Read the model definition and answer for the solid it produces. Units are mm, in the model's axes. A direction names the side the tool comes from. Coordinates: 2 decimals unless noted, no trailing zeros. Loops run counter-clockwise (first coordinate to the right, second up) from the corner with the lowest first, then second, coordinate; pieces in that order, holes last.
Q1. The mould has two halves that part along Z. Classify faces 1 (the face through (0, 0, 15)), 2 (the face through (-22.465, -1.617, -0.67)), 3 (the face through (0, -0.75, 9)), 4 (the face through (0, 9, -0.75)): pulls with the +Z half, pulls with the -Z half, needs draft (parallel to the pull), parting line crosses it, or undercut.
Q2. Which of the six approach directions +Z, -Z, +X, -X, +Y, -Y give full straight-line access (tool end or side, diameter ignored) to faces 5 (the face through (0.28, -6.6, 5.55)), 6 (the face through (0, -0.75, -9)), 7 (the face through (0.28, 5.54, 6.61))?
Q3. Section C-C (z = -3.5) is taken. Give the vertices of the cut face in (x, y), then the cut area to 3 significant figures.
Q4. Straight lines are drawn through the part: line 1 (Z direction, x = 12, y = -10.5); line 2 (Z direction, x = -9.5, y = -5.5); line 3 (Y direction, x = 1, z = 8.5). For each, find the intervals that lie inside material, in ascending order.
Q5. Flat-ended cylindrical pins translate along their axes: P1, Ø1.5, axis at y = 9.5, z = -7, coming from the +X side; P2, Ø6.5, axis at x = 1.5, y = -9, coming from the -Z side; P3, Ø4, axis at x = 3.5, y = -6, coming from the +Z side; P4, Ø14, axis at x = 3.5, y = 9, coming from the +Z side. Find the tip coordinate at first contact, or state that the pin passes through.
Q6. Section A-A (y = -3.75) is taken. Give the vertices of the cut face in (x, z), then the cut area to 3 significant figures.
Q7. Section D-D (z = -12) is taken. Give the vertices of the cut face in (x, y), then the cut area to 3 significant figures.
from build123d import *

# Parameters (mm, degrees)
F0_W          = 40
F0_H          = 15
F3_DEPTH      = 40.001
F4_R          = 1.75
F4_R_2        = 0.75
F6_DEPTH      = 5
F6_DEPTH_BACK = 80


with BuildPart() as f1:
    # F0 (on Top) → F1 (revolve)
    with BuildSketch(Plane.XY):
        with Locations((0, 7.5)):
            Rectangle(F0_W, F0_H)
    revolve(axis=Axis((0, 0, 0), (1, 0, 0)))

    # F2 (on face) → F3 (cut, through all)
    with BuildSketch(Plane.YZ.offset(20)):
        with BuildLine():
            ThreePointArc((1.651475323, -0.578903496), (1.7251930059, -0.2936138491), (1.75, 0))
            ThreePointArc((1.75, 0), (1.7236043316, 0.3028004429), (1.6452135906, 0.5964664628))
            ThreePointArc((1.6452135906, 0.5964664628), (1.6150017407, 0.6739950872), (1.5811388301, 0.75))
            ThreePointArc((1.5811388301, 0.75), (1.2374368671, 1.2374368671), (0.75, 1.5811388301))
            ThreePointArc((0.75, 1.5811388301), (0.6653812907, 1.618569658), (0.5789024703, 1.6514756825))
            ThreePointArc((0.5789024703, 1.6514756825), (0, 1.75), (-0.5789024703, 1.6514756825))
            ThreePointArc((-0.5789024703, 1.6514756825), (-0.6653812907, 1.618569658), (-0.75, 1.5811388301))
            ThreePointArc((-0.75, 1.5811388301), (-1.2374368671, 1.2374368671), (-1.5811388301, 0.75))
            ThreePointArc((-1.5811388301, 0.75), (-1.6150017407, 0.6739950872), (-1.6452135906, 0.5964664628))
            ThreePointArc((-1.6452135906, 0.5964664628), (-1.7499751665, 0.0093229166), (-1.651475323, -0.578903496))
            ThreePointArc((-1.651475323, -0.578903496), (-1.6185694514, -0.6653817934), (-1.5811388301, -0.75))
            ThreePointArc((-1.5811388301, -0.75), (-1.2374368671, -1.2374368671), (-0.75, -1.5811388301))
            ThreePointArc((-0.75, -1.5811388301), (-0.6739945857, -1.61500195), (-0.596465441, -1.6452139611))
            ThreePointArc((-0.596465441, -1.6452139611), (0, -1.75), (0.596465441, -1.6452139611))
            ThreePointArc((0.596465441, -1.6452139611), (0.6739945857, -1.61500195), (0.75, -1.5811388301))
            ThreePointArc((0.75, -1.5811388301), (1.2374368671, -1.2374368671), (1.5811388301, -0.75))
            ThreePointArc((1.5811388301, -0.75), (1.6185694514, -0.6653817934), (1.651475323, -0.578903496))
        make_face()
        with BuildLine():
            ThreePointArc((2.2125773299, 1.1638305544), (2.3080064679, 0.9607841298), (2.3848480035, 0.75))
            Line((2.3848480035, 0.75), (14.9812382666, 0.75))
            ThreePointArc((14.9812382666, 0.75), (13.8565778233, 5.7441492866), (11.118002457, 10.0692612126))
            Line((11.118002457, 10.0692612126), (2.2125773299, 1.1638305544))
        make_face()
        with BuildLine():
            ThreePointArc((2.3848480035, -0.75), (2.3113855708, -0.9526262348), (2.2207433968, -1.1481719234))
            Line((2.2207433968, -1.1481719234), (11.1293184453, -10.0567525048))
            ThreePointArc((11.1293184453, -10.0567525048), (13.8598053196, -5.7363574246), (14.9812382666, -0.75))
            Line((14.9812382666, -0.75), (2.3848480035, -0.75))
        make_face()
        with BuildLine():
            Line((10.0692543074, -11.1180087108), (1.1638291802, -2.2125780527))
            ThreePointArc((1.1638291802, -2.2125780527), (0.960783413, -2.3080067663), (0.75, -2.3848480035))
            Line((0.75, -2.3848480035), (0.75, -14.9812382666))
            ThreePointArc((0.75, -14.9812382666), (5.7441449835, -13.8565796071), (10.0692543074, -11.1180087108))
        make_face()
        with BuildLine():
            Line((-0.75, -14.9812382666), (-0.75, -2.3848480035))
            ThreePointArc((-0.75, -2.3848480035), (-0.960783413, -2.3080067663), (-1.1638291802, -2.2125780527))
            Line((-1.1638291802, -2.2125780527), (-10.0692543074, -11.1180087108))
            ThreePointArc((-10.0692543074, -11.1180087108), (-5.7441449835, -13.8565796071), (-0.75, -14.9812382666))
        make_face()
        with BuildLine():
            Line((-11.1293184453, -10.0567525048), (-2.2207433968, -1.1481719234))
            ThreePointArc((-2.2207433968, -1.1481719234), (-2.3113855708, -0.9526262348), (-2.3848480035, -0.75))
            Line((-2.3848480035, -0.75), (-14.9812382666, -0.75))
            ThreePointArc((-14.9812382666, -0.75), (-13.8598053196, -5.7363574246), (-11.1293184453, -10.0567525048))
        make_face()
        with BuildLine():
            ThreePointArc((-2.3848480035, 0.75), (-2.3080064679, 0.9607841298), (-2.2125773299, 1.1638305544))
            Line((-2.2125773299, 1.1638305544), (-11.118002457, 10.0692612126))
            ThreePointArc((-11.118002457, 10.0692612126), (-13.8565778233, 5.7441492866), (-14.9812382666, 0.75))
            Line((-14.9812382666, 0.75), (-2.3848480035, 0.75))
        make_face()
        with BuildLine():
            ThreePointArc((-1.1481705441, 2.2207441099), (-0.952625517, 2.3113858666), (-0.75, 2.3848480035))
            Line((-0.75, 2.3848480035), (-0.75, 14.9812382666))
            ThreePointArc((-0.75, 14.9812382666), (-5.7363531205, 13.859807101), (-10.0567455926, 11.1293246914))
            Line((-10.0567455926, 11.1293246914), (-1.1481705441, 2.2207441099))
        make_face()
        with BuildLine():
            ThreePointArc((0.75, 2.3848480035), (0.952625517, 2.3113858666), (1.1481705441, 2.2207441099))
            Line((1.1481705441, 2.2207441099), (10.0567455926, 11.1293246914))
            ThreePointArc((10.0567455926, 11.1293246914), (5.7363531205, 13.859807101), (0.75, 14.9812382666))
            Line((0.75, 14.9812382666), (0.75, 2.3848480035))
        make_face()
    extrude(amount=-F3_DEPTH, mode=Mode.SUBTRACT)

    # F4 (on face) → F6 (join, two sides)
    with BuildSketch(Plane(origin=(-20, 0, 0), x_dir=(0, -1, 0), z_dir=(-1, 0, 0))) as f6_sk:
        Circle(F4_R)
        Circle(F4_R_2, mode=Mode.SUBTRACT)
        Circle(F4_R_2)
    extrude(amount=F6_DEPTH)
    extrude(f6_sk.sketch, amount=-F6_DEPTH_BACK)


solid = f1.part
Numbers:
1. face 1: pulls with the +Z half
1. face 2: parting line crosses it
1. face 3: needs draft
1. face 4: undercut
2. face 5: +X, -X, -Y
2. face 6: -Z, +X, -X
2. face 7: +Z, +X, -X
3. outline: (-20, -4.57) - (20, -4.57) - (20, -2.45) - (-20, -2.45) - close; (-20, -0.75) - (20, -0.75) - (20, 0.75) - (-20, 0.75) - close; (-20, 2.45) - (20, 2.45) - (20, 4.57) - (-20, 4.57) - close
3. area: 230 mm2
4. line 1: z = -10.71 to -9.43, -0.75 to 0.75, 9.45 to 10.71
4. line 2: z = -6.55 to -4.43, -0.75 to 0.75, 4.45 to 6.57
4. line 3: y = -9.55 to -7.43, -0.75 to 0.75, 7.43 to 9.55
5. P1: passes through
5. P2: stops at z = -11.12
5. P3: stops at z = 9.07
5. P4: stops at z = 11.13
6. outline: (-20, -4.8) - (20, -4.8) - (20, -2.68) - (-20, -2.68) - close; (-20, -0.75) - (20, -0.75) - (20, 0.75) - (-20, 0.75) - close; (-20, 2.7) - (20, 2.7) - (20, 4.82) - (-20, 4.82) - close
6. area: 230 mm2
7. outline: (-20, -0.75) - (20, -0.75) - (20, 0.75) - (-20, 0.75) - close
7. area: 60.0 mm2
